Part model, mm, in its own coordinate system. Face numbers are marked on the shaded views. A direction names the side the tool comes from. Round coordinates to 2 decimals unless told otherwise and drop trailing zeros. Write each loop counter-clockwise with the first axis right and the second up, starting at its lowest first coordinate (ties: lowest second). Pieces come first, ordered by that corner, then holes.
Autodesk Fusion 360 part; units mm, degrees
sketch "Sketch1" plane through (0, 0, 0) normal (0, 0, 1) x (1, 0, 0)
  circle A0 centre (0, 0) radius 9.5
  circle A1 centre (0, 0) radius 12.5
  circle A2 centre (0, 0) radius 15
  dimension "d1" = 19
  dimension "d2" = 25
  dimension "d3" = 30
extrude "Extrude1" add sketch "Sketch1" along normal blind 2 contours A1 | A2
extrude "Extrude2" add sketch "Sketch1" along normal blind 14 contours A1
fillet "Fillet1" radius 2 1 edges at (-8.8571, 3.4353, 0)
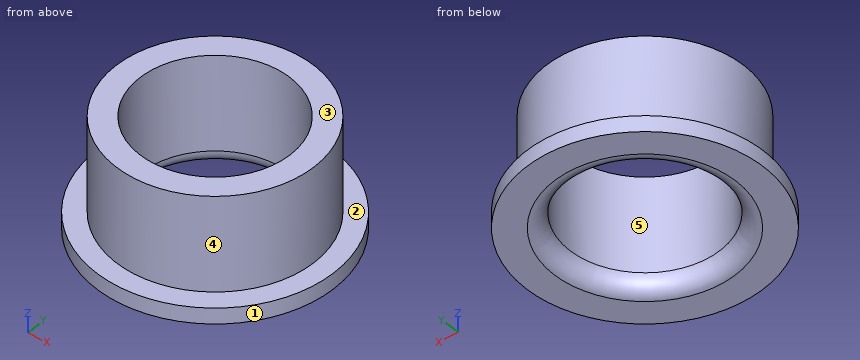
Q1. Mould opens along X. For the marked faces 3, 4 and 5 say: +X half, -X half, draft (parallel to the pull), parting line (faces both ways), or undercut.
Values follow:
face 3: draft
face 4: parting line
face 5: undercut
Q2. Drop flat-ended pins along their axis: pin 1 (6 mm diameter, centred on x = 1.5, y = -8, fed in from -Z); pin 2 (1.5 mm diameter, centred on x = 2.5, y = -9, fed in from -Z); pin 3 (1 mm diameter, centred on x = -6.5, z = 8, fed in from +Y); pin 4 (12 mm diameter, centred on x = 2, y = 1, fed in from +Z). Give the stop position or say it passes through.
Values follow:
pin 1: stops at z = 0.03
pin 2: stops at z = 0.58
pin 3: stops at y = 10.97
pin 4: passes through
Q3. Cut at C-C on z = 8.25. Write the cut outline in (x, y).
Values follow:
outline: circle Ø25 at (0, 0); hole circle Ø19 at (0, 0)
Q4. Wall check: L1, parallel to Y at x = 0, z = 10; L2, parallel to Z at x = 1.75, y = 13.5; L3, parallel to X at y = 2.5, z = 6.5. Give the ranges that are in metal, low to high.
Values follow:
L1: y = -12.5 to -9.5, 9.5 to 12.5
L2: z = 0 to 2
L3: x = -12.25 to -9.17, 9.17 to 12.25
Q5. Cut at D-D on z = 1.25. Write the cut outline in (x, y).
Values follow:
outline: circle Ø30 at (0, 0); hole circle Ø19.29 at (0, 0)
Q6. Which spindle directions (+Z, -Z, +X, -X, +Y, -Y) get a long thin tool onto all of the face, cutting with end or side? Do the marked faces 1 and 2. Say none if no direction does.
Values follow:
face 1: +Z, -Z
face 2: +Z
Q7. Cut at A-A on y = 0. Write the cut outline in (x, z).
Values follow:
outline: (-15, 0) - (-11.5, 0) arc R2 ccw to (-9.5, 2) - (-9.5, 14) - (-12.5, 14) - (-12.5, 2) - (-15, 2) - close; (9.5, 2) arc R2 ccw to (11.5, 0) - (15, 0) - (15, 2) - (12.5, 2) - (12.5, 14) - (9.5, 14) - close
